Verification items for the finished model (mm, model axes). A direction names the side the tool comes from. Coordinates: 2 decimals unless noted, no trailing zeros. Loops run counter-clockwise (first coordinate to the right, second up) from the corner with the lowest first, then second, coordinate; pieces in that order, holes last. Notation, with made-up numbers: (69.25, -33.5) -> (84.25, -33.5) arc R27 cw to (84.25, -2.5) -> close; hole circle Ø7 at (20, 45). An arc over 180 degrees is marked (long way). Write item = value, one per line.
```python
from build123d import *

# Parameters (mm, degrees)
SKETCH_1_R          = 3.625
EXTRUDE_1_DEPTH     = 16
SKETCH_2_R          = 3.625
EXTRUDE_3_DEPTH     = 3
EXTRUDE_4_DEPTH     = 42.25
SKETCH_4_R          = 11.5
SKETCH_4_R_2        = 1.75
CUT_EXTRUDE_1_DEPTH = 42.25
EXTRUDE_5_REACH     = 85.549
SKETCH_5_R          = 3.915
SKETCH_5_R_2        = 3.625
CUT_EXTRUDE_2_REACH = 85.549
CHAMFER_1_SIZE      = 0.5
CHAMFER_2_SIZE      = 1
CHAMFER_3_SIZE      = 5
SKETCH_7_W          = 19.912738871
SKETCH_7_H          = 22.903585025
CUT_EXTRUDE_3_DEPTH = 2
CHAMFER_4_SIZE      = 0.5


with BuildPart() as part:
    # Sketch 1 → Extrude 1 (new body)
    with BuildSketch(Plane(origin=(0, 0, 0), x_dir=(1, 0, 0), z_dir=(0, 1, 0))):
        with Locations(Location((0, 0, 0), (0, 0, 270))):
            Circle(SKETCH_1_R)
    extrude(amount=EXTRUDE_1_DEPTH)

    # Sketch 2 → Extrude 3 (add)
    # profile 1 of 15: a face of its own
    with BuildSketch(Plane(origin=(0, 16, 0), x_dir=(1, 0, 0), z_dir=(0, 1, 0))):
        with BuildLine():
            Line((52.7, 21.25), (12.7, 21.25))
            Line((12.7, 21.25), (12.7, 12.896511156))
            ThreePointArc((12.7, 12.896511156), (16.695508378, 6.990708119), (18.1, 0))
            ThreePointArc((18.1, 0), (16.695508378, -6.990708119), (12.7, -12.896511156))
            Line((12.7, -12.896511156), (12.7, -21.25))
            Line((12.7, -21.25), (52.7, -21.25))
            Line((52.7, -21.25), (52.7, 21.25))
        make_face()
    # profile 2 of 15: a face of its own
    with BuildSketch(Plane(origin=(0, 16, 0), x_dir=(1, 0, 0), z_dir=(0, 1, 0))):
        with BuildLine():
            ThreePointArc((18.1, 0), (16.695508378, 6.990708119), (12.7, 12.896511156))
            Line((12.7, 12.896511156), (12.7, 8.168231143))
            ThreePointArc((12.7, 8.168231143), (14.487580888, 4.256759331), (15.1, 0))
            ThreePointArc((15.1, 0), (14.487580888, -4.256759331), (12.7, -8.168231143))
            Line((12.7, -8.168231143), (12.7, -12.896511156))
            ThreePointArc((12.7, -12.896511156), (16.695508378, -6.990708119), (18.1, 0))
        make_face()
    # profile 3 of 15: a face of its own
    with BuildSketch(Plane(origin=(0, 16, 0), x_dir=(1, 0, 0), z_dir=(0, 1, 0))):
        with BuildLine():
            Line((12.7, 21.25), (10.1, 21.25))
            Line((10.1, 21.25), (10.1, 15.019986684))
            ThreePointArc((10.1, 15.019986684), (11.449335661, 14.018655889), (12.7, 12.896511156))
            Line((12.7, 12.896511156), (12.7, 21.25))
        make_face()
    # profile 4 of 15: a face of its own
    with BuildSketch(Plane(origin=(0, 16, 0), x_dir=(1, 0, 0), z_dir=(0, 1, 0))):
        with BuildLine():
            ThreePointArc((12.7, 12.896511156), (11.449335661, 14.018655889), (10.1, 15.019986684))
            Line((10.1, 15.019986684), (10.1, 11.22497216))
            ThreePointArc((10.1, 11.22497216), (11.501996192, 9.78335748), (12.7, 8.168231143))
            Line((12.7, 8.168231143), (12.7, 12.896511156))
        make_face()
    # profile 5 of 15: a face of its own
    with BuildSketch(Plane(origin=(0, 16, 0), x_dir=(1, 0, 0), z_dir=(0, 1, 0))):
        with BuildLine():
            ThreePointArc((12.7, -8.168231143), (11.501996192, -9.78335748), (10.1, -11.22497216))
            Line((10.1, -11.22497216), (10.1, -15.019986684))
            ThreePointArc((10.1, -15.019986684), (11.449335661, -14.018655889), (12.7, -12.896511156))
            Line((12.7, -12.896511156), (12.7, -8.168231143))
        make_face()
    # profile 6 of 15: a face of its own
    with BuildSketch(Plane(origin=(0, 16, 0), x_dir=(1, 0, 0), z_dir=(0, 1, 0))):
        with BuildLine():
            ThreePointArc((12.7, 8.168231143), (11.501996192, 9.78335748), (10.1, 11.22497216))
            Line((10.1, 11.22497216), (10.1, -11.22497216))
            ThreePointArc((10.1, -11.22497216), (11.501996192, -9.78335748), (12.7, -8.168231143))
            Line((12.7, -8.168231143), (12.7, 8.168231143))
        make_face()
    # profile 7 of 15: a face of its own
    with BuildSketch(Plane(origin=(0, 16, 0), x_dir=(1, 0, 0), z_dir=(0, 1, 0))):
        with BuildLine():
            ThreePointArc((15.1, 0), (14.487580888, 4.256759331), (12.7, 8.168231143))
            Line((12.7, 8.168231143), (12.7, -8.168231143))
            ThreePointArc((12.7, -8.168231143), (14.487580888, -4.256759331), (15.1, 0))
        make_face()
    # profile 8 of 15: a face of its own
    with BuildSketch(Plane(origin=(0, 16, 0), x_dir=(1, 0, 0), z_dir=(0, 1, 0))):
        with BuildLine():
            Line((10.1, -21.25), (12.7, -21.25))
            Line((12.7, -21.25), (12.7, -12.896511156))
            ThreePointArc((12.7, -12.896511156), (11.449335661, -14.018655889), (10.1, -15.019986684))
            Line((10.1, -15.019986684), (10.1, -21.25))
        make_face()
    # profile 9 of 15: a face of its own
    with BuildSketch(Plane(origin=(0, 16, 0), x_dir=(1, 0, 0), z_dir=(0, 1, 0))):
        with BuildLine():
            Line((10.1, 11.22497216), (10.1, 15.019986684))
            ThreePointArc((10.1, 15.019986684), (3.404020503, 17.777025747), (-3.836808066, 17.688665972))
            Line((-3.836808066, 17.688665972), (-5.119556865, 17.360879514))
            ThreePointArc((-5.119556865, 17.360879514), (-18.096837592, -0.3383329), (-4.467058756, -17.540107926))
            ThreePointArc((-4.467058756, -17.540107926), (3.085491781, -17.83507052), (10.1, -15.019986684))
            Line((10.1, -15.019986684), (10.1, -11.22497216))
            ThreePointArc((10.1, -11.22497216), (-15.1, 0), (10.1, 11.22497216))
        make_face()
    # profile 10 of 15: a face of its own
    with BuildSketch(Plane(origin=(0, 16, 0), x_dir=(1, 0, 0), z_dir=(0, 1, 0))):
        with BuildLine():
            ThreePointArc((10.1, -15.019986684), (3.085491781, -17.83507052), (-4.467058756, -17.540107926))
            Line((-4.467058756, -17.540107926), (10.1, -21.25))
            Line((10.1, -21.25), (10.1, -15.019986684))
        make_face()
    # profile 11 of 15: a face of its own
    with BuildSketch(Plane(origin=(0, 16, 0), x_dir=(1, 0, 0), z_dir=(0, 1, 0))):
        with BuildLine():
            Line((10.1, -11.22497216), (10.1, 11.22497216))
            ThreePointArc((10.1, 11.22497216), (-15.1, 0), (10.1, -11.22497216))
        make_face()
        with Locations(Location((0, 0, 0), (0, 0, 270))):
            Circle(SKETCH_2_R, mode=Mode.SUBTRACT)
    # profile 12 of 15: a face of its own
    with BuildSketch(Plane(origin=(0, 16, 0), x_dir=(1, 0, 0), z_dir=(0, 1, 0))):
        with Locations(Location((0, 0, 0), (0, 0, 270))):
            Circle(SKETCH_2_R)
    # profile 13 of 15: a face of its own
    with BuildSketch(Plane(origin=(0, 16, 0), x_dir=(1, 0, 0), z_dir=(0, 1, 0))):
        with BuildLine():
            Line((10.1, 15.019986684), (10.1, 21.25))
            Line((10.1, 21.25), (-3.836808066, 17.688665972))
            ThreePointArc((-3.836808066, 17.688665972), (3.404020503, 17.777025747), (10.1, 15.019986684))
        make_face()
    # profile 14 of 15: a face of its own
    with BuildSketch(Plane(origin=(0, 16, 0), x_dir=(1, 0, 0), z_dir=(0, 1, 0))):
        with BuildLine():
            ThreePointArc((12.7, 12.896511156), (11.449335661, 14.018655889), (10.1, 15.019986684))
            Line((10.1, 15.019986684), (10.1, 11.22497216))
            ThreePointArc((10.1, 11.22497216), (11.501996192, 9.78335748), (12.7, 8.168231143))
            Line((12.7, 8.168231143), (12.7, 12.896511156))
        make_face()
    # profile 15 of 15: a face of its own
    with BuildSketch(Plane(origin=(0, 16, 0), x_dir=(1, 0, 0), z_dir=(0, 1, 0))):
        with BuildLine():
            ThreePointArc((12.7, -8.168231143), (11.501996192, -9.78335748), (10.1, -11.22497216))
            Line((10.1, -11.22497216), (10.1, -15.019986684))
            ThreePointArc((10.1, -15.019986684), (11.449335661, -14.018655889), (12.7, -12.896511156))
            Line((12.7, -12.896511156), (12.7, -8.168231143))
        make_face()
    extrude(amount=EXTRUDE_3_DEPTH)

    # Sketch 3 → Extrude 4 (add)
    with BuildSketch(Plane(origin=(0, 19, 0), x_dir=(1, 0, 0), z_dir=(0, 1, 0))):
        with BuildLine():
            Line((12.7, 12.896511156), (12.7, 21.25))
            Line((12.7, 21.25), (10.1, 21.25))
            Line((10.1, 21.25), (10.1, 15.019986684))
            ThreePointArc((10.1, 15.019986684), (11.449335661, 14.018655889), (12.7, 12.896511156))
        make_face()
        with BuildLine():
            Line((12.7, 8.168231143), (12.7, 12.896511156))
            ThreePointArc((12.7, 12.896511156), (11.449335661, 14.018655889), (10.1, 15.019986684))
            Line((10.1, 15.019986684), (10.1, 11.22497216))
            ThreePointArc((10.1, 11.22497216), (11.501996192, 9.78335748), (12.7, 8.168231143))
        make_face()
        with BuildLine():
            Line((12.7, -12.896511156), (12.7, -8.168231143))
            ThreePointArc((12.7, -8.168231143), (11.501996192, -9.78335748), (10.1, -11.22497216))
            Line((10.1, -11.22497216), (10.1, -15.019986684))
            ThreePointArc((10.1, -15.019986684), (11.449335661, -14.018655889), (12.7, -12.896511156))
        make_face()
        with BuildLine():
            Line((12.7, -8.168231143), (12.7, 8.168231143))
            ThreePointArc((12.7, 8.168231143), (11.501996192, 9.78335748), (10.1, 11.22497216))
            Line((10.1, 11.22497216), (10.1, -11.22497216))
            ThreePointArc((10.1, -11.22497216), (11.501996192, -9.78335748), (12.7, -8.168231143))
        make_face()
        with BuildLine():
            Line((12.7, -21.25), (12.7, -12.896511156))
            ThreePointArc((12.7, -12.896511156), (11.449335661, -14.018655889), (10.1, -15.019986684))
            Line((10.1, -15.019986684), (10.1, -21.25))
            Line((10.1, -21.25), (12.7, -21.25))
        make_face()
    extrude(amount=EXTRUDE_4_DEPTH)

    # Sketch 4 → Cut-Extrude 1 (cut)
    with BuildSketch(Plane.ZY.offset(-10.1)):
        with Locations((0, 40.125)):
            Circle(SKETCH_4_R)
        with Locations((-15.5, 55.533823529)):
            Circle(SKETCH_4_R_2)
        with Locations((15.5, 55.533823529)):
            Circle(SKETCH_4_R_2)
        with Locations((15.5, 24.716176471)):
            Circle(SKETCH_4_R_2)
        with Locations((-15.5, 24.716176471)):
            Circle(SKETCH_4_R_2)
    extrude(amount=-CUT_EXTRUDE_1_DEPTH, mode=Mode.SUBTRACT)

    # Sketch 5 → Extrude 5 (add, up to next)
    with BuildSketch(Plane.XZ, mode=Mode.PRIVATE) as extrude_5_sk1:
        with Locations(Location((0, 0, 0), (0, 0, 270))):
            Circle(SKETCH_5_R)
        Circle(SKETCH_5_R_2, mode=Mode.SUBTRACT)
    extrude_5_tool1 = extrude(extrude_5_sk1.sketch, amount=-EXTRUDE_5_REACH, mode=Mode.PRIVATE) - part.part
    add(extrude_5_tool1.solids().sort_by_distance((0, 0, 3.804267))[0])

    # Sketch 6 → Cut-Extrude 2 (cut, up to next)
    with BuildSketch(Plane.XZ, mode=Mode.PRIVATE) as cut_extrude_2_sk1:
        with BuildLine():
            Line((-1.516575089, -2.05), (1.516575089, -2.05))
            ThreePointArc((1.516575089, -2.05), (0, 2.55), (-1.516575089, -2.05))
        make_face()
    cut_extrude_2_tool1 = extrude(cut_extrude_2_sk1.sketch, amount=-CUT_EXTRUDE_2_REACH, mode=Mode.PRIVATE) & part.part
    add(cut_extrude_2_tool1.solids().sort_by_distance((0, 0, 0.119895))[0], mode=Mode.SUBTRACT)

    # Chamfer 1
    chamfer_1_edges = [part.edges().sort_by_distance(p)[0] for p in [
        (12.7, 24.716176471, -17.25),
        (10.1, 24.716176471, -17.25),
        (12.7, 24.716176471, 13.75),
        (10.1, 24.716176471, 13.75),
        (12.7, 55.533823529, 13.75),
        (10.1, 55.533823529, 13.75),
        (12.7, 55.533823529, -17.25),
        (10.1, 55.533823529, -17.25),
        (12.7, 40.125, -11.5),
        (10.1, 40.125, -11.5),
        (2.816470622, 19, 19.395053963),
        (0, 0, 3.915),
        (0, 19, -2.05),
        (0, 19, 2.55),
        (0, 0, -2.05),
        (0, 0, 2.55),
        (-18.096837592, 19, 0.3383329),
        (2.490221568, 19, -19.305439757),
    ]]
    chamfer(chamfer_1_edges, length=CHAMFER_1_SIZE)

    # Chamfer 2
    chamfer_2_edges = [part.edges().sort_by_distance(p)[0] for p in [
        (10.1, 19, 5.2997e-05),
    ]]
    chamfer(chamfer_2_edges, length=CHAMFER_2_SIZE)

    # Chamfer 3
    chamfer_3_edges = [part.edges().sort_by_distance(p)[0] for p in [
        (11.4, 61.25, 21.25),
        (11.4, 61.25, -21.25),
        (52.7, 17.5, 21.25),
        (52.7, 17.5, -21.25),
    ]]
    chamfer(chamfer_3_edges, length=CHAMFER_3_SIZE)

    # Sketch 7 → Cut-Extrude 3 (cut)
    with BuildSketch(Plane.XZ):
        with Locations((2.581888661, -2.951492916)):
            Rectangle(SKETCH_7_W, SKETCH_7_H)
    extrude(amount=-CUT_EXTRUDE_3_DEPTH, mode=Mode.SUBTRACT)

    # Chamfer 4
    chamfer_4_edges = [part.edges().sort_by_distance(p)[0] for p in [
        (0, 2, 2.55),
        (0, 2, 3.915),
        (0, 2, -2.05),
    ]]
    chamfer(chamfer_4_edges, length=CHAMFER_4_SIZE)


solid = part.part
```
1) Sectioned sample at B-B, the plane y = 17.5. Record the cut outline in (x, z).
Ans:
outline = (-5.12, -17.36) -> (10.1, -21.25) -> (47.7, -21.25) -> (52.7, -16.25) -> (52.7, 16.25) -> (47.7, 21.25) -> (10.1, 21.25) -> (-4.47, 17.54) arc R18.1 ccw to start; hole (-1.52, -2.05) -> (1.52, -2.05) arc R2.55 ccw (long way) to start
2) Release check for a two-part mould opening along Z. For faces 1 (the face through (0, 2, -3)), 2 (the face through (12, 27, 21.25)), 3 (the face through (11.39, 25.24, 17.17)), 4 (the face through (11.4, 28.9, -2.5)) record: pulls with the +Z half, pulls with the -Z half, needs draft (parallel to the pull), parting line crosses it, or undercut.
Ans:
face_1 = needs draft
face_2 = pulls with the +Z half
face_3 = undercut
face_4 = undercut
3) Depth check by flat-ended pin: pin 1 Ø4 at (y, z) = (55.53, -15.5) entering from -X; pin 2 Ø4.5 at (x, z) = (0, 0) entering from -Y; pin 3 Ø10 at (y, z) = (54, 16) entering from +X; pin 4 Ø14 at (y, z) = (40.125, 0) entering from +X. Enter the tip coordinate at first touch or a pass-through.
Ans:
pin_1 = 10.35
pin_2 = 2.3
pin_3 = 12.7
pin_4 = through
4) Sectioned sample at A-A, the plane z = 0. Count the separate pieces of the cut face and the enclosed holes in it, plus the area to 3 significant figures.
Ans:
separate_pieces = 3
enclosed_holes = 0
area = 284 mm2
5) Material ranges on line 1 (X direction, y = 6, z = 0) (3 decimals); line 2 (Y direction, x = 11, z = 15); line 3 (Y direction, x = 28, z = -11), recorded low to high.
Ans:
line_1 = -3.915 to -2.55, 2.55 to 3.915
line_2 = 16 to 23.04, 26.39 to 53.86, 57.21 to 61.25
line_3 = 16 to 19
6) Tool access check on faces 5 (the face through (3.412, 18.865, 19.17)), 6 (the face through (-4, 19, 0)), 7 (the face through (12.7, 30, -9)). Record the directions out of +Z, -Z, +X, -X, +Y, -Y that give a thin tool (end or side, any length) a straight path to the whole face; none if there is none.
Ans:
face_5 = +Z, -X, +Y
face_6 = +Z, -Z, -X, +Y
face_7 = +Z, -Z, +X, +Y
7) Sectioned sample at D-D, the plane x = 17.5. Record the cut outline in (y, z).
Ans:
outline = (16, -21.25) -> (19, -21.25) -> (19, 21.25) -> (16, 21.25) -> close
8) Sectioned sample at C-C, the plane x = 0. Record the cut outline in (y, z) (3 decimals).
Ans:
outline = (2, -3.415) -> (2.5, -3.915) -> (16, -3.915) -> (16, -18.669) -> (18.5, -18.669) -> (19, -18.153) -> (19, -2.55) -> (18.5, -2.05) -> (2.5, -2.05) -> (2, -2.55) -> close; (2, 3.05) -> (2.5, 2.55) -> (18.5, 2.55) -> (19, 3.05) -> (19, 18.162) -> (18.5, 18.678) -> (16, 18.678) -> (16, 3.915) -> (2.5, 3.915) -> (2, 3.415) -> close
